```python
from build123d import *

# Parameters (mm, degrees)
CUT_EXTRUDE1_DEPTH = 12.065
SKETCH4_R          = 2.5527
CUT_EXTRUDE2_DEPTH = 7.35
CIRPATTERN1_COUNT  = 4


with BuildPart() as part:
    # Sketch2 → Revolve1 (revolve)
    with BuildSketch(Plane(origin=(0, 0, 0), x_dir=(0, 0, -1), z_dir=(1, 0, 0))):
        with BuildLine():
            Line((6, 34), (-6, 34))
            Line((-6, 34), (-6.127, 33.873))
            Line((-6.127, 33.873), (-9.525, 33.873))
            Line((-9.525, 33.873), (-9.525, 44.45))
            Line((-9.525, 44.45), (9.525, 44.45))
            ThreePointArc((9.525, 44.45), (18.725516989, 40.158239998), (24.415, 31.75))
            Line((24.415, 31.75), (24.415, 19.05))
            Line((24.415, 19.05), (14.89, 19.05))
            Line((14.89, 19.05), (14.89, 21.59))
            ThreePointArc((14.89, 21.59), (12.286179285, 27.876179285), (6, 30.48))
            Line((6, 30.48), (6, 34))
        make_face()
    revolve(axis=Axis((0, 0, 0), (0, 0, 1)))

    # Sketch3 → Cut-Extrude1 (cut)
    with BuildSketch(Plane.XY.offset(-6)):
        Polygon((5.499261314, 25.4), (2.749630657, 30.1625), (-2.749630657, 30.1625), (-5.499261314, 25.4), (-2.749630657, 20.6375), (2.749630657, 20.6375), align=None)
    cut_extrude1 = extrude(amount=-CUT_EXTRUDE1_DEPTH, mode=Mode.SUBTRACT)

    # Sketch4 → Cut-Extrude2 (cut, through all)
    with BuildSketch(Plane.XY.offset(-18.065)):
        with Locations((0, 25.4)):
            Circle(SKETCH4_R)
    cut_extrude2 = extrude(amount=-CUT_EXTRUDE2_DEPTH, mode=Mode.SUBTRACT)

    # CirPattern1: Cut-Extrude1, Cut-Extrude2 ×4 about axis
    cirpattern1_axis = Axis((0, 0, 0), (0, 0, 1))
    for i in range(1, CIRPATTERN1_COUNT):
        add(cut_extrude1.rotate(cirpattern1_axis, i * 360 / CIRPATTERN1_COUNT), mode=Mode.SUBTRACT)
        add(cut_extrude2.rotate(cirpattern1_axis, i * 360 / CIRPATTERN1_COUNT), mode=Mode.SUBTRACT)


solid = part.part
```
For this review, take the finished solid that the model builds, in its own axes (mm). A direction names the side the tool comes from. Coordinates: 2 decimals unless noted, no trailing zeros. Write each loop counter-clockwise with the first axis right and the second up, starting at its lowest first coordinate (ties: lowest second). Pieces come first, ordered by that corner, then holes. Notation, with made-up numbers: (46, 24) - (66, 24) arc R14 cw to (66, 33) - close; hole circle Ø11 at (-30.75, 78). An arc over 180 degrees is marked (long way). Put each result on its own line as item: value.
1. Add section B-B, the plane y = 0. Count the separate pieces of the cut face and the enclosed holes in it, then the cut area to 3 significant figures.
Values found:
separate pieces: 4
enclosed holes: 0
area: 819 mm²
2. Machinability: for faces 1 (the flat face through (-4.144, 23.052, -16.347)), 2 (the cylindrical face through (-1.372, -27.552, -21.196)), which of the approach directions +Z, -Z, +X, -X, +Y, -Y give a long, thin tool a straight path to every point of the face, cutting with its end or side? Answer none if there is none.
Values found:
face 1: +Z
face 2: +Z, -Z
3. Add section A-A, the plane z = -21. Give the boundary of the cut face in (x, y), then the cut area to 3 significant figures.
Values found:
outline: circle Ø75.71 at (0, 0); hole circle Ø5.11 at (-25.4, 0); hole circle Ø38.1 at (0, 0); hole circle Ø5.11 at (0, -25.4); hole circle Ø5.11 at (0, 25.4); hole circle Ø5.11 at (25.4, 0)
area: 3,280 mm²
4. Wall thickness on probe 1 along X at (y, z) = (1, 8); probe 2 along Y at (x, z) = (0, -21); probe 3 along Y at (x, z) = (0, -19.25): over which ranges is each line inside the solid? List them lowest first.
Values found:
probe 1: -44.44 to -33.86, 33.86 to 44.44
probe 2: -37.86 to -27.95, -22.85 to -19.05, 19.05 to 22.85, 27.95 to 37.86
probe 3: -39.69 to -27.95, -22.85 to -19.05, 19.05 to 22.85, 27.95 to 39.69
5. Add section D-D, the plane z = -2. Give the boundary of the cut face in (x, y), then the cut area to 3 significant figures.
Values found:
outline: circle Ø88.9 at (0, 0); hole circle Ø68 at (0, 0)
area: 2,580 mm²
6. Mouldability with a two-part tool opening along Z and no side actions: class faces 3 (the cylindrical face through (-28.67, 18.28, 0.08)), 4 (the flat face through (-8, 18, -14.89)), 5 (the flat face through (-28, -4, -15)) as released by +Z, released by -Z, zero draft, split by the parting line, or undercut.
Values found:
face 3: undercut
face 4: released by +Z
face 5: zero draft
7. For pin 1 (4 mm diameter, centred on y = -32.5, z = -17, fed in from -X); pin 2 (3 mm diameter, centred on x = 25, z = 1, fed in from +Y); pin 3 (6 mm diameter, centred on x = -0.5, z = -13.5, fed in from -Y), all flat-tipped, find the tip position at first contact; note any pin that passes through.
Values found:
pin 1: x = -28.76
pin 2: y = 37.73
pin 3: y = -44.26
